Read the model definition and answer for the solid it produces. Units are mm, in the model's axes. Face numbers are marked on the shaded views. A direction names the side the tool comes from. Round coordinates to 2 decimals unless told otherwise and drop trailing zeros. Write each loop counter-clockwise with the first axis right and the second up, starting at its lowest first coordinate (ties: lowest second). Pieces come first, ordered by that corner, then holes. Notation, with made-up numbers: (24, 76.5) -> (36, 76.5) arc R23 ccw to (36, 85.5) -> close; hole circle Ø9 at (-26.75, 6.5). An arc over 180 degrees is marked (long way). Return JSON: item names as keys, results as strings.
Autodesk Inventor part; units mm, degrees
ref_plane "YZ Plane" through (0, 0, 0) normal (1, 0, 0) x (0, 1, 0)
ref_plane "XZ Plane" through (0, 0, 0) normal (0, 1, 0) x (-1, 0, 0)
ref_plane "XY Plane" through (0, 0, 0) normal (0, 0, 1) x (1, 0, 0)
sketch "Sketch1" plane through (0, 0, 0) normal (1, 0, 0) x (0, 1, 0)
  arc A0 (20, 7.5) -> (20, 47.5) centre (20, 27.5) ccw
  line L0 (5, 55) -> (0, 55)
  line L1 (0, 55) -> (0, 0)
  line L2 (0, 0) -> (5, 0)
  circle A1 centre (20, 27.5) radius 20 construction
  circle A2 centre (20, 15) radius 1.5
  circle A3 centre (20, 40) radius 1.5
  circle A4 centre (20, 27.5) radius 7.5
  line L3 (20, 47.5) -> (5, 47.5)
  line L4 (5, 47.5) -> (5, 55)
  line L5 (20, 7.5) -> (5, 7.5)
  line L6 (5, 7.5) -> (5, 0)
  dimension "d0" = 20
  dimension "d3" = 5
  dimension "d5" = 3
  dimension "d6" = 3
  dimension "d7" = 25
  dimension "d8" = 12.5
  dimension "d9" = 15
  dimension "d30" = 55
extrude "Extrusion1" add sketch "Sketch1" along normal blind 5
sketch "Sketch2" plane through (5, 0, 0) normal (1, 0, 0) x (0, 0, -1)
  line L0 (-55, 5) -> (-55, 0)
  line L1 (-47.5, 20) -> (-47.5, 5)
  line L2 (-55, 5) -> (-47.5, 5)
  line L3 (-47.5, 5) -> (-47.5, 20)
  line L4 (-55, 0) -> (0, 0)
  line L5 (-55, 0) -> (0, 0)
  line L6 (-55, 0) -> (-55, 5)
  circle A0 centre (-27.5, 20) radius 20
  arc A1 (-7.5, 20) -> (-47.5, 20) centre (-27.5, 20) ccw
  line L7 (0, 0) -> (0, 5)
  line L8 (0, 0) -> (0, 5)
  line L9 (0, 5) -> (-7.5, 5)
  line L10 (-7.5, 5) -> (-7.5, 20)
  line L11 (-7.5, 5) -> (-7.5, 20)
  point P0 (-7.5, 20)
  point P1 (-27.5, 0)
extrude "Extrusion2" add sketch "Sketch2" along normal blind 20 contours L2 L1 A0 L4 L0 | A0 L10 L9 L7 L4
chamfer "Chamfer1" distance 2 angle 45 2 edges at (12.5, 5, 7.5) (12.5, 5, 47.5)
sketch "Sketch3" plane through (0, 5, 0) normal (0, 1, 0) x (1, 0, 0)
  circle A0 centre (6.25, -2.75) radius 1.5
  circle A1 centre (18.75, -2.75) radius 1.5
  circle A2 centre (6.25, -52.25) radius 1.5
  circle A3 centre (18.75, -52.25) radius 1.5
  line L0 (0, -55) -> (25, -55)
  line L1 (0, -49.5) -> (25, -49.5)
  line L2 (0, 0) -> (25, 0)
  line L3 (25, -5.5) -> (0, -5.5)
  line L4 (0, -49.5) -> (0, -55)
  line L5 (25, -49.5) -> (25, -55)
  dimension "d20" = 3
  dimension "d21" = 2.75
  dimension "d22" = 2.75
  dimension "d23" = 2.75
  dimension "d24" = 2.75
  dimension "d25" = 6.25
  dimension "d26" = 6.25
  dimension "d27" = 12.5
extrude "Extrusion3" cut sketch "Sketch3" against normal through all contours A0 | A1 | A2 | A3
equation "\"d21\" = d22"
equation "\"d23\" = d24"
equation "\"d25\" = 0.5 * d27"
equation "\"d26\" = d25"
properties part number "motor mount"
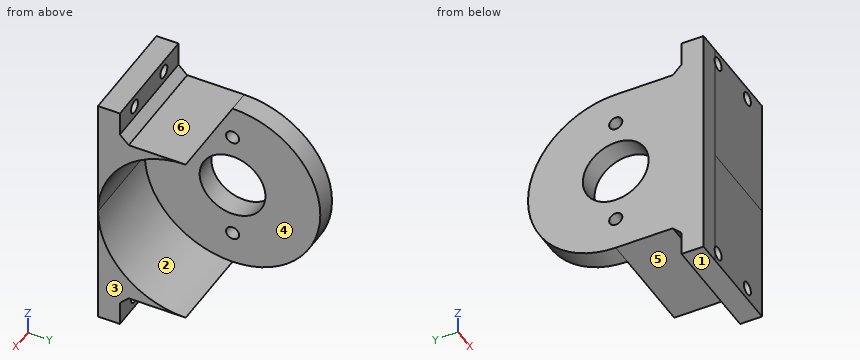
Item 1: A tool of negligible diameter and unlimited length cuts with its end or side. For the marked faces 4, 5 and 6, from which of +Z, -Z, +X, -X, +Y, -Y can it reach the whole face along a straight path? Write none if from no direction.
Worked answers:
{"face 4": "+X, +Y", "face 5": "-Z, +X, -X, +Y", "face 6": "+Z, +X, -X, +Y"}
Item 2: Section A-A (z = 52.25) is taken. Give the vertices of the cut face in (x, y), then the cut area to 3 significant figures.
Worked answers:
{"outline": "(0, 0) -> (4.75, 0) -> (4.75, 5) -> (0, 5) -> close; (7.75, 0) -> (17.25, 0) -> (17.25, 5) -> (7.75, 5) -> close; (20.25, 0) -> (25, 0) -> (25, 5) -> (20.25, 5) -> close", "area": "95.0 mm2"}
Item 3: Section D-D (x = 2) is taken. Give the vertices of the cut face in (y, z), then the cut area to 3 significant figures.
Worked answers:
{"outline": "(0, 0) -> (5, 0) -> (5, 5.5) -> (7, 7.5) -> (20, 7.5) arc R20 ccw to (20, 47.5) -> (7, 47.5) -> (5, 49.5) -> (5, 55) -> (0, 55) -> close; hole circle Ø15 at (20, 27.5); hole circle Ø3 at (20, 15); hole circle Ø3 at (20, 40)", "area": "1,320 mm2"}
Item 4: Flat-ended cylindrical pins translate along their axes: pin 1 (6.5 mm diameter, centred on x = 12.5, y = 16, fed in from +Z); pin 2 (1 mm diameter, centred on y = 26.5, z = 45, fed in from +X); pin 3 (3 mm diameter, centred on x = 17, z = 53, fed in from +Y). Find the tip coordinate at first contact, or state that the pin passes through.
Worked answers:
{"pin 1": "stops at z = 47.5", "pin 2": "stops at x = 5", "pin 3": "stops at y = 5"}
Item 5: For a pull along Z with two mould halves and no side action, classify the marked faces 1, 2 and 3 as released by +Z, released by -Z, zero draft, split by the parting line, or undercut.
Worked answers:
{"face 1": "released by -Z", "face 2": "undercut", "face 3": "zero draft"}
Item 6: Straight lines are drawn through the part: L1, parallel to Z at x = 2.6, y = 20; L2, parallel to X at y = 1.2, z = 2.75; L3, parallel to X at y = 24, z = 38.5. For each, find the intervals that lie inside material, in ascending order. Write a range as [from, to].
Worked answers:
{"L1": "z = [7.5, 13.5], [16.5, 20], [35, 38.5], [41.5, 47.5]", "L2": "x = [0, 4.75], [7.75, 17.25], [20.25, 25]", "L3": "x = [0, 5]"}
